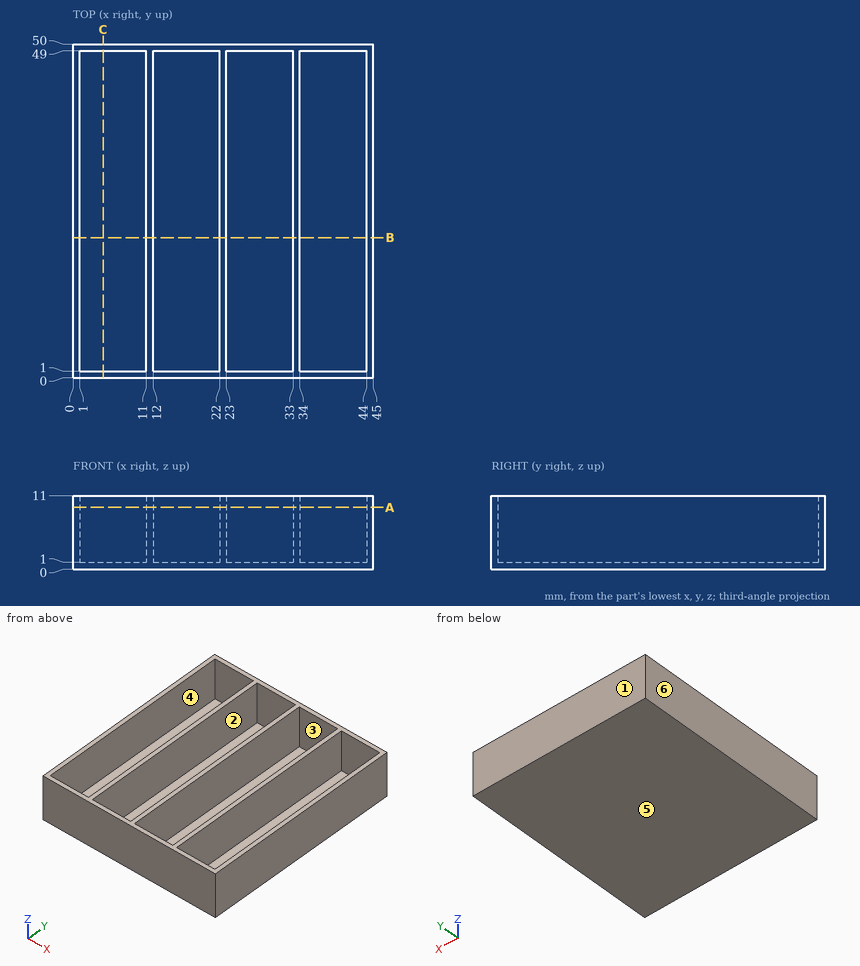
The drawing under review shows one solid part. Ordinate dimensions are in mm from its lowest x, y, z. A direction names the side the tool comes from. Give positions to 0.01 mm unless a question says otherwise; leave off trailing zeros. Order: outer loops, then holes, each group sorted by start corner. A loop starts at its lowest first (then second) coordinate and runs counter-clockwise, first axis right, second up. Notation, with made-up numbers: M -6.75,-39 L 22.25,-39 A25 ccw 22.25,-8 Z; hole C 55,18 d6. An arc over 180 degrees is marked long. Answer in a Markdown table with one row per item. Add a question column.
1. For pin 1 Ø5 at (x, y) = (38, 26) entering from +Z, flat-tipped, find the tip position at first contact; note if it passes through.
2. To check wall thickness, follow line 1 along X through (y, z) = (3, 6.5); line 2 along Y through (x, z) = (18, 4); line 3 along Z through (x, y) = (8, 47). State the ranges of each line that lie inside material, in increasing order.
3. Add section B-B on y = 21. State the section outline as (x, z) points, plus the area to 3 significant figures.
4. Add section C-C on x = 4.5. State the section outline as (y, z) points.
5. Machinability: for the marked faces 1 and 2, which of the approach directions +Z, -Z, +X, -X, +Y, -Y give a long, thin tool a straight path to every point of the face, cutting with its end or side? Answer none if there is none.
6. Add section A-A on z = 9.25. State the section outline as (x, y) points, plus the area to 3 significant figures.
7. Mouldability with a two-part tool opening along X and no side actions: class the marked faces 3, 4, 5 and 6 as released by +X, released by -X, zero draft, split by the parting line, or undercut.
The answers:
| question | item | result |
|---|---|---|
| 1 | pin 1 | z = 1 |
| 2 | line 1 | 0 to 1, 11 to 12, 22 to 23, 33 to 34, 44 to 45 |
| 2 | line 2 | 0 to 1, 49 to 50 |
| 2 | line 3 | 0 to 1 |
| 3 | outline | M 0,0 L 45,0 L 45,11 L 44,11 L 44,1 L 34,1 L 34,11 L 33,11 L 33,1 L 23,1 L 23,11 L 22,11 L 22,1 L 12,1 L 12,11 L 11,11 L 11,1 L 1,1 L 1,11 L 0,11 Z |
| 3 | area | 95.0 mm2 |
| 4 | outline | M 0,0 L 50,0 L 50,11 L 49,11 L 49,1 L 1,1 L 1,11 L 0,11 Z |
| 5 | face 1 | +Z, -Z, +X, -X, +Y |
| 5 | face 2 | +Z |
| 6 | outline | M 0,0 L 45,0 L 45,50 L 0,50 Z; hole M 1,1 L 11,1 L 11,49 L 1,49 Z; hole M 12,1 L 22,1 L 22,49 L 12,49 Z; hole M 23,1 L 33,1 L 33,49 L 23,49 Z; hole M 34,1 L 44,1 L 44,49 L 34,49 Z |
| 6 | area | 330 mm2 |
| 7 | face 3 | undercut |
| 7 | face 4 | undercut |
| 7 | face 5 | zero draft |
| 7 | face 6 | released by -X |
